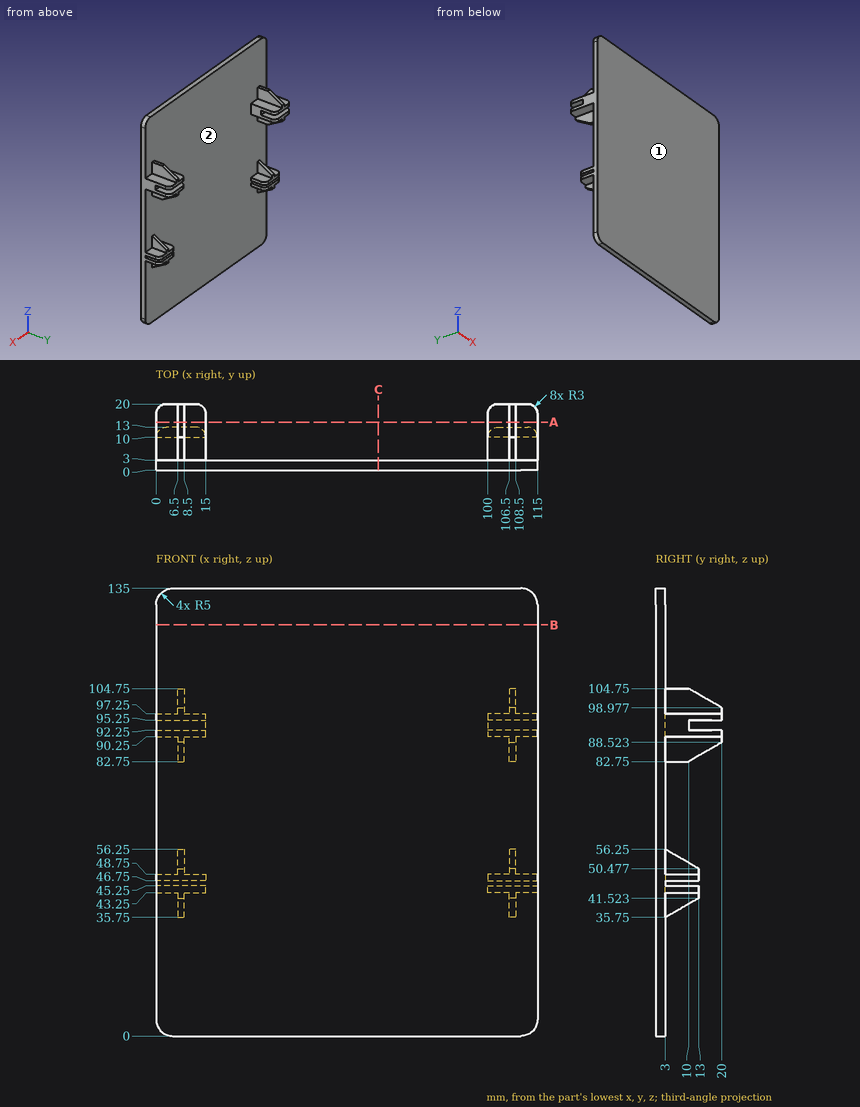
Study the drawing (mm; zero at the part's minimum x, y, z) and answer. Round coordinates to 2 decimals unless told otherwise and drop trailing zeros. Write each loop counter-clockwise with the first axis right and the second up, starting at its lowest first coordinate (ties: lowest second). Pieces come first, ordered by that corner, then holes.
1) A cutting plane is placed at B-B (z = 124). Give the vertices of the cut face in (x, y).
2) A cutting plane is placed at A-A (y = 14.5). Give the number of separate pieces and of enclosed holes in the cut face, plus the area to 3 significant figures.
3) The mould has two halves that part along X. Classify the marked faces 1 and 2: pulls with the +X half, pulls with the -X half, needs draft (parallel to the pull), parting line crosses it, or undercut.
4) Straight lines are drawn through the part: line 1 (Z direction, x = 103.5, y = 7.25); line 2 (Z direction, x = 101.5, y = 19.25); line 3 (X direction, y = 17, z = 88). For each, find the intervals that lie inside material, in ascending order.
5) A cutting plane is placed at C-C (x = 67). Give the vertices of the cut face in (y, z).
6) Given pin 1 Ø1.6 at (x, y) = (107.5, 6.5) entering from +Z; pin 2 Ø5 at (x, y) = (12, 10.5) entering from +Z; pin 3 Ø1 at (x, y) = (7.5, 5.5) entering from -Z (1 decimal), each flat-ended and moving along its own axis, determine where each tip first touches the part or whether it passes through.
Completed:
1. outline: (0, 0) - (115, 0) - (115, 3) - (0, 3) - close
2. separate pieces: 4
2. enclosed holes: 0
2. area: 159 mm2
3. face 1: needs draft
3. face 2: undercut
4. line 1: z = 43.25 to 45.25, 46.75 to 48.75, 90.25 to 97.25
4. line 2: z = 90.25 to 92.25, 95.25 to 97.25
4. line 3: x = 6.5 to 8.5, 106.5 to 108.5
5. outline: (0, 0) - (3, 0) - (3, 135) - (0, 135) - close
6. pin 1: stops at z = 104.75
6. pin 2: stops at z = 97.25
6. pin 3: stops at z = 36.9
